from build123d import *

# Parameters (mm, degrees)
SKETCH1_W              = 203.2
SKETCH1_H              = 254
BOSS_EXTRUDE1_DEPTH    = 3.175
SKETCH2_R              = 3.3734375
CUT_EXTRUDE1_DEPTH     = 326.294206258
F_10_32_TAPPED_HOLE1_D = 4.0386


with BuildPart() as part:
    # Sketch1 → Boss-Extrude1 (new body)
    with BuildSketch(Plane(origin=(0, 0, 0), x_dir=(1, 0, 0), z_dir=(0, 1, 0))):
        with Locations((101.6, 127)):
            Rectangle(SKETCH1_W, SKETCH1_H)
    extrude(amount=BOSS_EXTRUDE1_DEPTH)

    # Sketch2 → Cut-Extrude1 (cut, through all)
    with BuildSketch(Plane(origin=(0, 3.175, 0), x_dir=(1, 0, 0), z_dir=(0, 1, 0))):
        with Locations(Location((190.5, 203.2, 0), (0, 0, 270))):
            Circle(SKETCH2_R)
        with Locations(Location((12.7, 203.2, 0), (0, 0, 270))):
            Circle(SKETCH2_R)
        with Locations(Location((12.7, 50.8, 0), (0, 0, 270))):
            Circle(SKETCH2_R)
        with Locations(Location((190.5, 50.8, 0), (0, 0, 270))):
            Circle(SKETCH2_R)
    extrude(amount=-CUT_EXTRUDE1_DEPTH, mode=Mode.SUBTRACT)

    # #10-32 Tapped Hole1 (through all)
    with Locations(Plane(origin=(0, 3.175, 0), x_dir=(1, 0, 0), z_dir=(0, 1, 0))):
        with Locations((172.72, 25.4), (172.72, 93.98), (30.48, 25.4), (30.48, 93.98)):
            Hole(F_10_32_TAPPED_HOLE1_D / 2)


solid = part.part
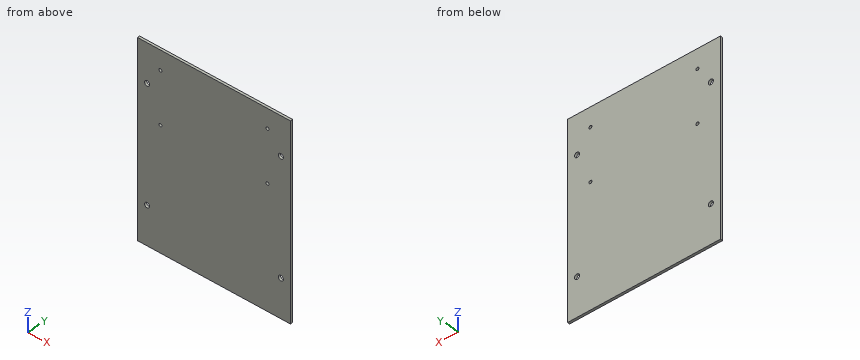
Build history of the part. All positions in model axes, mm. Coordinates: 2 decimals unless noted, no trailing zeros. Write each loop counter-clockwise with the first axis right and the second up, starting at its lowest first coordinate (ties: lowest second). Pieces come first, ordered by that corner, then holes. Notation, with made-up numbers: (-18.75, -33) -> (0.25, -33) arc R25 ccw to (0.25, -3) -> close; hole circle Ø4 at (-28, 72). An arc over 180 degrees is marked (long way). Use CSV: the item, a comma, the result in double quotes. Start each with the question number.
Q1. Drill centre lines: probe 1 along X at (y, z) = (1, -25.4); probe 2 along Z at (x, y) = (172.72, 0.7); probe 3 along X at (y, z) = (1.15, -50.8). Where is each one in solid material? Low to high.
Q2. Flat gauge pins, fed straight in: pin 1 Ø3.5 at (x, z) = (172.72, -93.98) entering from -Y; pin 2 Ø1.5 at (x, z) = (147, -132.5) entering from -Y. Where does each tip first touch, or does it go through?
Q3. Cut at A-A, the plane x = 12.7. List the corners of the cut face in (y, z) (3 decimals), then the cut area to 3 significant figures.
Checked values:
1,probe 1,"x = 0 to 28.46, 32.5 to 170.7, 174.74 to 203.2"
1,probe 2,"z = -254 to -96, -91.96 to -27.42, -23.38 to 0"
1,probe 3,"x = 0 to 9.33, 16.07 to 187.13, 193.87 to 203.2"
2,pin 1,"passes through"
2,pin 2,"stops at y = 0"
3,outline,"(0, -254) -> (3.175, -254) -> (3.175, -206.573) -> (0, -206.573) -> close; (0, -199.827) -> (3.175, -199.827) -> (3.175, -54.173) -> (0, -54.173) -> close; (0, -47.427) -> (3.175, -47.427) -> (3.175, 0) -> (0, 0) -> close"
3,area,"764 mm²"
